The listing builds one solid part. Answer for the finished solid, in the listing's coordinates (mm). Face numbers are marked on the shaded views. A direction names the side the tool comes from. Coordinates: 2 decimals unless noted, no trailing zeros. Loops run counter-clockwise (first coordinate to the right, second up) from the corner with the lowest first, then second, coordinate; pieces in that order, holes last. Notation, with made-up numbers: (87, 78) - (98, 78) arc R12 ccw to (98, 93) - close; hole circle Ø7 at (45, -5.5). An arc over 180 degrees is marked (long way). Write each question's results on one line, items separated by ' | '. Start each with the question number.
(1) Find section C-C on z = -30. Determine the outline of the cut face in (x, y), then the cut area to 3 significant figures.
(2) Given pin 1 Ø1.5 at (x, z) = (37, -37) entering from +Y; pin 2 Ø2.5 at (x, z) = (5.5, -37) entering from +Y; pin 3 Ø6 at (x, z) = (26, -9.5) entering from +Y, each flat-ended and moving along its own axis, determine where each tip first touches the part or whether it passes through.
(3) For the marked faces 1 and 2, determine the directions among +Z, -Z, +X, -X, +Y, -Y from which every point of the face is accessible in a straight line to the end or side of a thin tool.
(4) Find section D-D on x = 29.5. Determine the outline of the cut face in (y, z).
(5) Find section A-A on z = -21. Determine the outline of the cut face in (x, y).
(6) Find section B-B on x = 36.5. Determine the outline of the cut face in (y, z), then the cut area to 3 significant figures.
(7) Consider line 1 (X direction, y = 37.05, z = -5.5); line 2 (Z direction, x = 36.5, y = 36.95); line 3 (Y direction, x = 10, z = -12). Determine where each line is inside the solid, lowest interval first. Write a range as from..to.
from build123d import *

# Parameters (mm, degrees)
BOSS_EXTRUDE1_DEPTH = 40
SKETCH2_R           = 11
BOSS_EXTRUDE2_DEPTH = 2
SKETCH3_R           = 2.5
BOSS_EXTRUDE3_DEPTH = 15
SKETCH4_R           = 1.5
CUT_EXTRUDE1_DEPTH  = 5


with BuildPart() as part:
    # Sketch1 → Boss-Extrude1 (new body)
    with BuildSketch(Plane(origin=(0, 0, 0), x_dir=(1, 0, 0), z_dir=(0, 1, 0))):
        with BuildLine():
            Line((3, 0), (39, 0))
            ThreePointArc((39, 0), (41.121320344, 0.878679656), (42, 3))
            Line((42, 3), (42, 39))
            ThreePointArc((42, 39), (41.121320344, 41.121320344), (39, 42))
            Line((39, 42), (3, 42))
            ThreePointArc((3, 42), (0.878679656, 41.121320344), (0, 39))
            Line((0, 39), (0, 3))
            ThreePointArc((0, 3), (0.878679656, 0.878679656), (3, 0))
        make_face()
    extrude(amount=BOSS_EXTRUDE1_DEPTH)

    # Sketch2 → Boss-Extrude2 (add)
    with BuildSketch(Plane(origin=(0, 40, 0), x_dir=(1, 0, 0), z_dir=(0, 1, 0))):
        with Locations((21, 21)):
            Circle(SKETCH2_R)
    extrude(amount=BOSS_EXTRUDE2_DEPTH)

    # Sketch3 → Boss-Extrude3 (add)
    with BuildSketch(Plane(origin=(0, 42, 0), x_dir=(1, 0, 0), z_dir=(0, 1, 0))):
        with Locations((21, 21)):
            Circle(SKETCH3_R)
    extrude(amount=BOSS_EXTRUDE3_DEPTH)

    # Sketch4 → Cut-Extrude1 (cut)
    with BuildSketch(Plane(origin=(0, 40, 0), x_dir=(1, 0, 0), z_dir=(0, 1, 0))):
        with Locations((5.5, 36.5)):
            Circle(SKETCH4_R)
        with Locations((36.5, 36.5)):
            Circle(SKETCH4_R)
        with Locations((36.5, 5.5)):
            Circle(SKETCH4_R)
        with Locations((5.5, 5.5)):
            Circle(SKETCH4_R)
    extrude(amount=-CUT_EXTRUDE1_DEPTH, mode=Mode.SUBTRACT)


solid = part.part
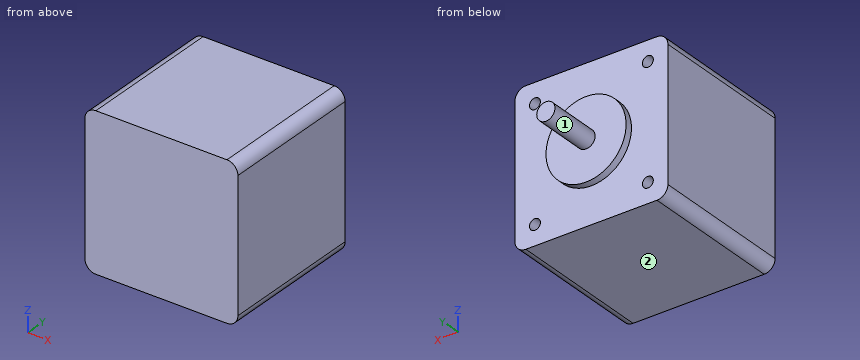
Values:
1) outline: (0, 0) - (42, 0) - (42, 40) - (27.32, 40) - (27.32, 42) - (14.68, 42) - (14.68, 40) - (0, 40) - close | area: 1,710 mm²
2) pin 1: stops at y = 35 | pin 2: stops at y = 40 | pin 3: stops at y = 42
3) face 1: +Y | face 2: -Z, +X, -X, +Y, -Y
4) outline: (0, -42) - (40, -42) - (40, -27.98) - (42, -27.98) - (42, -14.02) - (40, -14.02) - (40, 0) - (0, 0) - close
5) outline: (0, 0) - (42, 0) - (42, 40) - (32, 40) - (32, 42) - (23.5, 42) - (23.5, 57) - (18.5, 57) - (18.5, 42) - (10, 42) - (10, 40) - (0, 40) - close
6) outline: (0, -42) - (40, -42) - (40, -38) - (35, -38) - (35, -35) - (40, -35) - (40, -7) - (35, -7) - (35, -4) - (40, -4) - (40, 0) - (0, 0) - close | area: 1,650 mm²
7) line 1: x = 0..4, 7..35, 38..42 | line 2: z = -42..-38, -35..-7, -4..0 | line 3: y = 0..40
